```python
from build123d import *

# Parameters (mm, degrees)
SKETCH_1_W          = 35
SKETCH_1_H          = 26
EXTRUDE_1_DEPTH     = 26
SKETCH_3_W          = 13
SKETCH_3_H          = 13
SKETCH_3_H_2        = 7
CUT_EXTRUDE_1_DEPTH = 43


with BuildPart() as part:
    # 草圖1 → 填料-伸長1 (new body)
    with BuildSketch(Plane.XY):
        Rectangle(SKETCH_1_W, SKETCH_1_H)
    extrude(amount=EXTRUDE_1_DEPTH)

    # 草圖3 → 除料-伸長1 (cut)
    with BuildSketch(Plane.ZY.offset(17.5)):
        with Locations((13, 6.5)):
            Rectangle(SKETCH_3_W, SKETCH_3_H)
        with Locations((13, -9.5)):
            Rectangle(SKETCH_3_W, SKETCH_3_H_2)
    extrude(amount=-CUT_EXTRUDE_1_DEPTH, mode=Mode.SUBTRACT)


solid = part.part
```
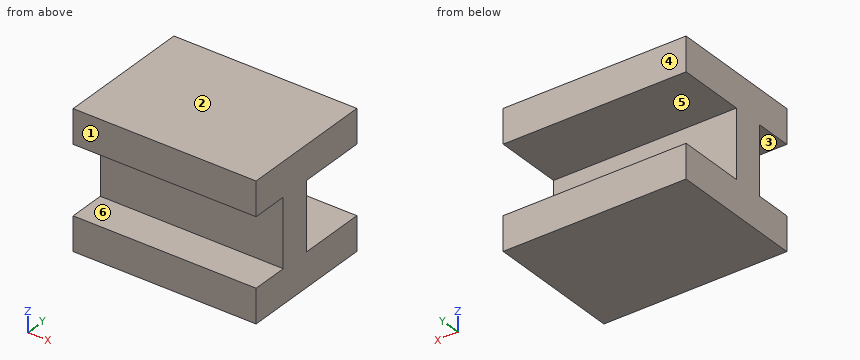
For this review, take the finished solid that the model builds, in its own axes (mm). Face numbers are marked on the shaded views. A direction names the side the tool comes from. Coordinates: 2 decimals unless noted, no trailing zeros. Write each loop counter-clockwise with the first axis right and the second up, starting at its lowest first coordinate (ties: lowest second). Pieces come first, ordered by that corner, then holes. Notation, with made-up numbers: (-14.5, 31.25) - (17.5, 31.25) arc R31 cw to (17.5, 65.25) - close; hole circle Ø3 at (-5, 66.5). An arc over 180 degrees is marked (long way). Answer in a Markdown table with one row per item. Add a question column.
Q1. We need section A-A, the plane y = 6. State the section outline as (x, z) points.
Q2. We need section B-B, the plane x = -14. State the section outline as (y, z) points, and give its area (3 significant figures).
Q3. Tool access review of the marked faces 4, 5 and 6: name each direction out of +Z, -Z, +X, -X, +Y, -Y from which nothing blocks a thin tool from reaching the whole face with its end or side.
Q4. We need section C-C, the plane z = 12.25. State the section outline as (x, y) points.
Q5. For P1, Ø6, axis at x = -0.5, y = 5.5, coming from the -Z side; P2, Ø6.5, axis at x = -1.5, z = 13.5, coming from the +Y side, all flat-tipped, find the tip position at first contact; note any pin that passes through.
Q6. Draft analysis for pull direction Z (two halves, no side actions). For the marked faces 1, 2 and 3, state which applies: +Z half, -Z half, draft (parallel to the pull), parting line (faces both ways), or undercut.
Q7. For probe 1 along Z at (x, y) = (-9, 0.75); probe 2 along Y at (x, z) = (-14.5, 8.25), list the stretches that pass through material, from the lowest coordinate up.
Answer list:
| question | item | result |
|---|---|---|
| 1 | outline | (-17.5, 0) - (17.5, 0) - (17.5, 6.5) - (-17.5, 6.5) - close; (-17.5, 19.5) - (17.5, 19.5) - (17.5, 26) - (-17.5, 26) - close |
| 2 | outline | (-13, 0) - (13, 0) - (13, 6.5) - (0, 6.5) - (0, 19.5) - (13, 19.5) - (13, 26) - (-13, 26) - (-13, 19.5) - (-6, 19.5) - (-6, 6.5) - (-13, 6.5) - close |
| 2 | area | 416 mm2 |
| 3 | face 4 | +Z, -Z, +X, -X, +Y |
| 3 | face 5 | +X, -X, +Y |
| 3 | face 6 | +X, -X, -Y |
| 4 | outline | (-17.5, -6) - (17.5, -6) - (17.5, 0) - (-17.5, 0) - close |
| 5 | P1 | stops at z = 0 |
| 5 | P2 | stops at y = 0 |
| 6 | face 1 | draft |
| 6 | face 2 | +Z half |
| 6 | face 3 | undercut |
| 7 | probe 1 | z = 0 to 6.5, 19.5 to 26 |
| 7 | probe 2 | y = -6 to 0 |
